Answer from the drawing. Dimensions are ordinates in mm from the lowest x, y and z of the part. A direction names the side the tool comes from. Coordinates: 2 decimals unless noted, no trailing zeros. Write each loop counter-clockwise with the first axis right and the second up, starting at its lowest first coordinate (ties: lowest second). Pieces come first, ordered by that corner, then holes.
(1) Straight lines are drawn through the part: line 1 (Y direction, x = 17, z = 10); line 2 (Y direction, x = 35.5, z = 7.75); line 3 (X direction, y = 4.75, z = 1.5) (1 decimal). For each, find the intervals that lie inside material, in ascending order.
(2) The part is cut by section C-C on x = 17.5. Determine the outline of the cut face in (y, z), plus the area to 3 significant figures.
(3) For a pull along X with two mould halves and no side action, classify the marked faces 1, 2 and 3 as +X half, -X half, draft (parallel to the pull), parting line (faces both ways), or undercut.
(4) The part is cut by section A-A on y = 2.5. Give the number of separate pieces and of enclosed holes in the cut face.
(5) Given P1, Ø2, axis at x = 27, z = 6.5, coming from the -Y side (1 decimal); P2, Ø8, axis at x = 34.5, y = 4, coming from the +Z side; P3, Ø8, axis at x = 33.5, z = 16.5, coming from the -Y side, each flat-ended and moving along its own axis, determine where each tip first touches the part or whether it passes through.
(6) Which of the six approach directions +Z, -Z, +X, -X, +Y, -Y give full straight-line access (tool end or side, diameter ignored) to the marked faces 4, 5, 6, 7 and 8?
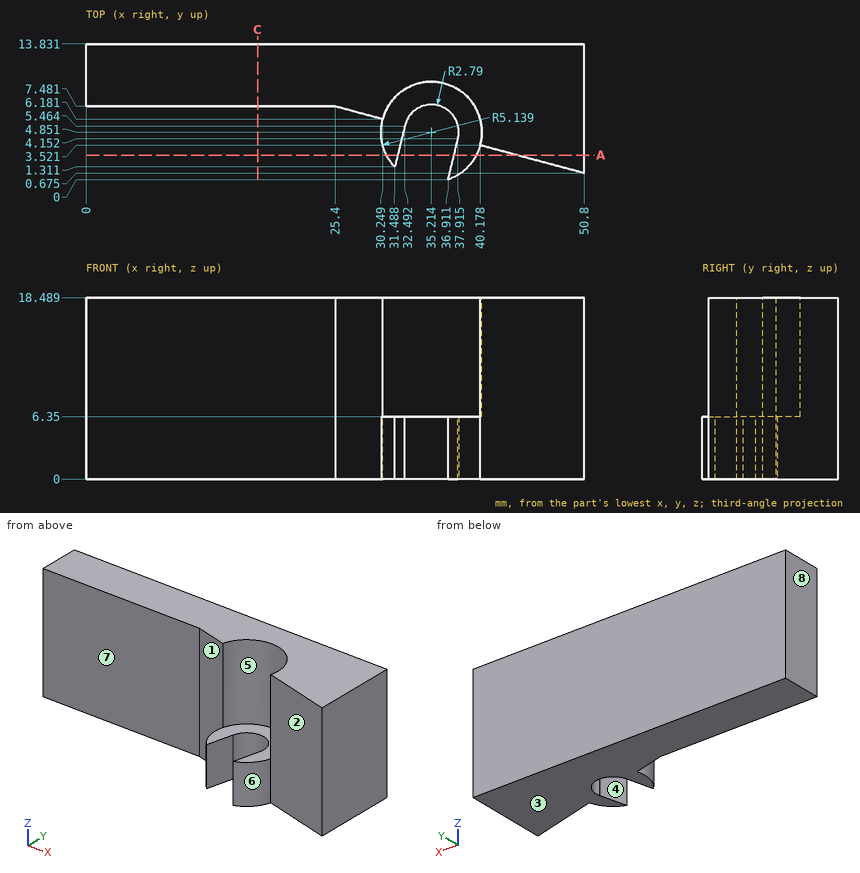
Model answer:
1. line 1: y = 7.48 to 13.83
1. line 2: y = 9.98 to 13.83
1. line 3: x = 30.1 to 32.3, 38 to 50.8
2. outline: (7.48, 0) - (13.83, 0) - (13.83, 18.49) - (7.48, 18.49) - close
2. area: 117 mm2
3. face 1: -X half
3. face 2: undercut
3. face 3: draft
4. separate pieces: 3
4. enclosed holes: 0
5. P1: stops at y = 6.8
5. P2: stops at z = 6.35
5. P3: stops at y = 6.18
6. face 4: +Z, -Z
6. face 5: +Z
6. face 6: +Z, -Z, -Y
6. face 7: +Z, -Z, -X, -Y
6. face 8: +Z, -Z, -X, +Y, -Y
